from build123d import *

# Parameters (mm, degrees)
F1_W     = 104
F1_H     = 104
F2_DEPTH = 3
F3_R     = 5


with BuildPart() as f2:
    # F1 (on Top) → F2 (new body)
    with BuildSketch(Plane.XY):
        Rectangle(F1_W, F1_H)
        Polygon((28, -43), (28, -40), (-28, -40), (-28, -43), (-40, -43), (-40, -49), (-43, -49), (-43, -43), (-49, -43), (-49, -40), (-43, -40), (-43, -28), (-40, -28), (-40, 28), (-43, 28), (-43, 40), (-49, 40), (-49, 43), (-43, 43), (-43, 49), (-40, 49), (-40, 43), (-40, 40), (40, 40), (40, 43), (40, 49), (43, 49), (43, 43), (49, 43), (49, 40), (43, 40), (43, 28), (40, 28), (40, -28), (43, -28), (43, -40), (49, -40), (49, -43), (43, -43), (43, -49), (40, -49), (40, -43), align=None, mode=Mode.SUBTRACT)
        Polygon((28, -40), (40, -40), (40, -28), (40, 28), (40, 40), (-40, 40), (-40, 28), (-40, -28), (-40, -40), (-28, -40), align=None)
    extrude(amount=F2_DEPTH)

    # F3
    f3_edges = [f2.edges().sort_by_distance(p)[0] for p in [
        (-52, -52, 1.5),
        (-52, 52, 1.5),
        (52, -52, 1.5),
        (52, 52, 1.5),
    ]]
    fillet(f3_edges, radius=F3_R)


solid = f2.part
CAD build for the part. Positions are in the model's coordinates, mm. A direction names the side the tool comes from. Coordinates: 2 decimals unless noted, no trailing zeros. Loops run counter-clockwise (first coordinate to the right, second up) from the corner with the lowest first, then second, coordinate; pieces in that order, holes last. Notation, with made-up numbers: (66, -10.5) - (79, -10.5) arc R24 ccw to (79, 5.5) - close; hole circle Ø6 at (-20.5, 8.5). An arc over 180 degrees is marked (long way). Write item = value, one per line. Start each with the question number.
Q1. Cut at B-B, the plane z = 2.3. Give the number of separate pieces and of enclosed holes in the cut face, then the cut area to 3 significant figures.
Q2. Pull direction X, two halves, no side cores. Call faces 1 (the cylindrical face through (-51, 50, 2)), 2 (the flat face through (46, 43, 1)), 3 (the flat face through (-1, 52, 1)): pulls with the +X half, pulls with the -X half, needs draft (parallel to the pull), parting line crosses it, or undercut.
Q3. Which spindle directions (+Z, -Z, +X, -X, +Y, -Y) get a long thin tool onto all of the face, cutting with end or side? Do faces 4 (the flat face through (52, -1, 1)), 5 (the flat face through (40, -46, 1)). Say none if no direction does.
Q4. Cut at A-A, the plane y = 33.5. List the corners of the cut face in (x, z), then the cut area to 3 significant figures.
Q5. Drill centre lines: L1, parallel to X at y = -41.5, z = 0.55; L2, parallel to Y at x = -44.5, z = 0.8. Where is each one in solid material? Low to high.
Computed:
q1.separate_pieces = 1
q1.enclosed_holes = 4
q1.area = 10,400 mm²
q2.face_1 = pulls with the -X half
q2.face_2 = undercut
q2.face_3 = needs draft
q3.face_4 = +Z, -Z, +X, +Y, -Y
q3.face_5 = +Z, -Z
q4.outline = (-52, 0) - (-43, 0) - (-43, 3) - (-52, 3) - close; (-40, 0) - (40, 0) - (40, 3) - (-40, 3) - close; (43, 0) - (52, 0) - (52, 3) - (43, 3) - close
q4.area = 294 mm²
q5.L1 = -52 to -49, -28 to 28, 49 to 52
q5.L2 = -52 to -43, -40 to 40, 43 to 52
